The listing builds one solid part. Answer for the finished solid, in the listing's coordinates (mm). Face numbers are marked on the shaded views. A direction names the side the tool comes from. Round coordinates to 2 decimals unless told otherwise and drop trailing zeros. Order: outer loops, then holes, each group sorted by start corner. A loop starts at its lowest first (then second) coordinate and runs counter-clockwise, first axis right, second up. Notation, with made-up numbers: (50.5, 44.25) - (76.5, 44.25) arc R9 cw to (76.5, 55.25) - close; hole circle Ø4 at (88, 43.5). An arc over 180 degrees is marked (long way). One line per item, written item: value. Start each with the question number.
1. Section B-B, the plane y = 3.25 is taken. Give the vertices of the cut face in (x, z).
2. For a pull along X with two mould halves and no side action, classify the marked faces 1, 2 and 3 as released by +X, released by -X, zero draft, split by the parting line, or undercut.
3. Straight lines are drawn through the part: line 1 (X direction, y = 6.75, z = 0); line 2 (Y direction, x = 15.5, z = 7); line 3 (X direction, y = 7.75, z = 6). For each, find the intervals that lie inside material, in ascending order.
4. A tool of negligible diameter and unlimited length cuts with its end or side. For the marked faces 4 and 5, from which of +Z, -Z, +X, -X, +Y, -Y can it reach the whole face along a straight path? Write none if from no direction.
5. Section A-A, the plane z = 0 is taken. Give the vertices of the cut face in (x, y), then the cut area to 3 significant figures.
6. Flat-ended cylindrical pins translate along their axes: P1, Ø2, axis at y = 6.5, z = 10.5, coming from the -X side; P2, Ø3, axis at x = -7, y = 6.5, coming from the +Z side; P3, Ø1.5, axis at x = -1, y = 6.5, coming from the +Z side; P4, Ø1, axis at x = 1.5, z = -25, coming from the -Y side. Find the tip coordinate at first contact, or state that the pin passes through.
from build123d import *

# Parameters (mm, degrees)
SKETCH1_R           = 31.5
BOSS_EXTRUDE1_DEPTH = 15
SKETCH2_R           = 22.5
CUT_EXTRUDE1_DEPTH  = 13
SKETCH3_R           = 12.6
SKETCH3_R_2         = 2.5
CUT_EXTRUDE2_DEPTH  = 13
FILLET1_R           = 7


with BuildPart() as part:
    # Sketch1 → Boss-Extrude1 (new body)
    with BuildSketch(Plane(origin=(0, 0, 0), x_dir=(1, 0, 0), z_dir=(0, 1, 0))):
        with Locations(Location((0, 0, 0), (0, 0, 270))):
            Circle(SKETCH1_R)
    extrude(amount=BOSS_EXTRUDE1_DEPTH)

    # Sketch2 → Cut-Extrude1 (cut)
    with BuildSketch(Plane(origin=(0, 15, 0), x_dir=(1, 0, 0), z_dir=(0, 1, 0))):
        with Locations(Location((0, 0, 0), (0, 0, 270))):
            Circle(SKETCH2_R)
    extrude(amount=-CUT_EXTRUDE1_DEPTH, mode=Mode.SUBTRACT)

    # Sketch3 → Cut-Extrude2 (cut)
    with BuildSketch(Plane.XZ):
        with Locations(Location((0, 0, 0), (0, 0, 270))):
            Circle(SKETCH3_R)
        with Locations(Location((0, 20, 0), (0, 0, 270))):
            Circle(SKETCH3_R_2)
        with Locations(Location((0, -20, 0), (0, 0, 270))):
            Circle(SKETCH3_R_2)
    extrude(amount=-CUT_EXTRUDE2_DEPTH, mode=Mode.SUBTRACT)

    # Fillet1
    fillet1_edges = [part.edges().sort_by_distance(p)[0] for p in [
        (0, 0, -31.5),
    ]]
    fillet(fillet1_edges, radius=FILLET1_R)


solid = part.part
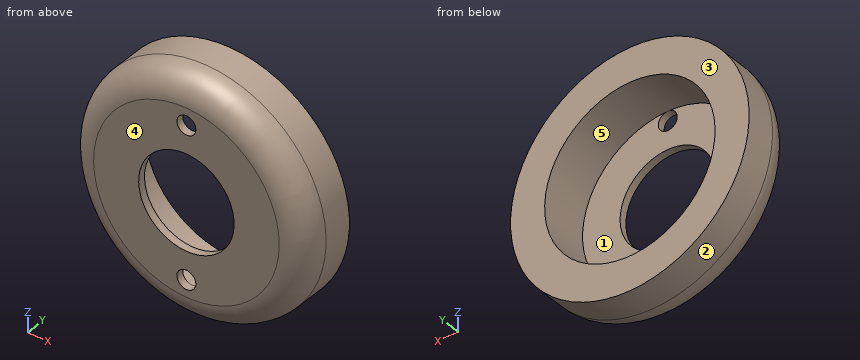
Answer list:
1. outline: circle Ø60.82 at (0, 0); hole circle Ø45 at (0, 0)
2. face 1: undercut
2. face 2: split by the parting line
2. face 3: zero draft
3. line 1: x = -31.5 to -22.5, 22.5 to 31.5
3. line 2: y = 0 to 2
3. line 3: x = -30.92 to -21.69, 21.69 to 30.92
4. face 4: +Z, -Z, +X, -X, -Y
4. face 5: +Y
5. outline: (-31.5, 7) arc R7 ccw to (-24.5, 0) - (-12.6, 0) - (-12.6, 2) - (-22.5, 2) - (-22.5, 15) - (-31.5, 15) - close; (12.6, 0) - (24.5, 0) arc R7 ccw to (31.5, 7) - (31.5, 15) - (22.5, 15) - (22.5, 2) - (12.6, 2) - close
5. area: 289 mm²
6. P1: stops at x = -30.02
6. P2: stops at z = 31.01
6. P3: stops at z = 31.5
6. P4: stops at y = 0
